```python
from build123d import *

# Parameters (mm, degrees)
SKETCH1_W           = 63.5
SKETCH1_H           = 48.26
BOSS_EXTRUDE1_DEPTH = 6.35
SKETCH2_R           = 3.683
CUT_EXTRUDE1_DEPTH  = 4.318
SKETCH3_R           = 2.159
CUT_EXTRUDE2_DEPTH  = 4.318
SKETCH5_W           = 46.99
SKETCH5_H           = 6.35
CUT_EXTRUDE3_DEPTH  = 2.032
SKETCH4_R           = 1.905
CUT_EXTRUDE4_DEPTH  = 14.732


with BuildPart() as part:
    # Sketch1 → Boss-Extrude1 (new body)
    with BuildSketch(Plane(origin=(0, 0, 0), x_dir=(1, 0, 0), z_dir=(0, 1, 0))):
        Rectangle(SKETCH1_W, SKETCH1_H)
    extrude(amount=-BOSS_EXTRUDE1_DEPTH)

    # Sketch2 → Cut-Extrude1 (cut)
    with BuildSketch(Plane(origin=(0, 0, 0), x_dir=(1, 0, 0), z_dir=(0, 1, 0))):
        with Locations((-19.05, 11.43)):
            Circle(SKETCH2_R)
    cut_extrude1 = extrude(amount=-CUT_EXTRUDE1_DEPTH, mode=Mode.SUBTRACT)

    # Sketch3 → Cut-Extrude2 (cut)
    with BuildSketch(Plane(origin=(0, -4.318, 0), x_dir=(1, 0, 0), z_dir=(0, 1, 0))):
        with Locations((-19.05, 11.43)):
            Circle(SKETCH3_R)
    cut_extrude2 = extrude(amount=-CUT_EXTRUDE2_DEPTH, mode=Mode.SUBTRACT)

    # Sketch5 → Cut-Extrude3 (cut)
    with BuildSketch(Plane.XZ.offset(6.35)):
        with Locations((8.255, 0)):
            Rectangle(SKETCH5_W, SKETCH5_H)
    extrude(amount=-CUT_EXTRUDE3_DEPTH, mode=Mode.SUBTRACT)

    # Sketch4 → Cut-Extrude4 (cut)
    with BuildSketch(Plane(origin=(0, 0, 0), x_dir=(1, 0, 0), z_dir=(0, 1, 0))):
        with Locations((-13.208, -19.558)):
            Circle(SKETCH4_R)
        with Locations((-13.208, 19.442)):
            Circle(SKETCH4_R)
        with Locations((24.638, -19.558)):
            Circle(SKETCH4_R)
        with Locations((24.638, 19.442)):
            Circle(SKETCH4_R)
    extrude(amount=-CUT_EXTRUDE4_DEPTH, mode=Mode.SUBTRACT)

    # Mirror1: Cut-Extrude1, Cut-Extrude2 across plane
    add(cut_extrude1.mirror(Plane.XY), mode=Mode.SUBTRACT)
    add(cut_extrude2.mirror(Plane.XY), mode=Mode.SUBTRACT)


solid = part.part
```
Model file for the job. Use its own axes, mm. A direction names the side the tool comes from. Coordinates: 2 decimals unless noted, no trailing zeros. Order: outer loops, then holes, each group sorted by start corner. A loop starts at its lowest first (then second) coordinate and runs counter-clockwise, first axis right, second up. Notation, with made-up numbers: M 5.25,74 L 24.25,74 A25 ccw 24.25,96 Z; hole C -35.75,4 d1. An arc over 180 degrees is marked long. Answer as CSV lines item,"result".
(1) Flat gauge pins, fed straight in: pin 1 (3 mm diameter, centred on x = 24.638, z = 19.558, fed in from -Y); pin 2 (3 mm diameter, centred on x = 3, z = 0.5, fed in from -Y); pin 3 (2 mm diameter, centred on y = -5.5, z = 1, fed in from +X). Where does each tip first touch, or does it go through?
Geometry says:
pin 1,"passes through"
pin 2,"stops at y = -4.32"
pin 3,"stops at x = -15.24"
(2) Band-saw the part on C-C, the plane z = -2.5. List the corners of the cut face in (x, y), then the cut area to 3 significant figures.
Geometry says:
outline,"M -31.75,-6.35 L -15.24,-6.35 L -15.24,-4.32 L 31.75,-4.32 L 31.75,0 L -31.75,0 Z"
area,"308 mm2"
(3) Band-saw the part on D-D, the plane y = -5.5. List the corners of the cut face in (x, z) (3 decimals), then the cut area to 3 significant figures.
Geometry says:
outline,"M -31.75,-24.13 L 31.75,-24.13 L 31.75,-3.175 L -15.24,-3.175 L -15.24,3.175 L 31.75,3.175 L 31.75,24.13 L -31.75,24.13 Z; hole C -19.05,-11.43 d4.318; hole C -19.05,11.43 d4.318; hole C -13.208,-19.442 d3.81; hole C -13.208,19.558 d3.81; hole C 24.638,-19.442 d3.81; hole C 24.638,19.558 d3.81"
area,"2,690 mm2"
(4) 3-axis set-ups, long thin cutter, end or side, ignore diameter. For faces 1 (the flat face through (-31.75, -3, 0)), 2 (the flat face through (8, -5, -3.175)), 3 (the cylindrical face through (-15.648, -2.129, 10.019)): which of +Z, -Z, +X, -X, +Y, -Y reach the whole face in a straight line?
Geometry says:
face 1,"+Z, -Z, -X, +Y, -Y"
face 2,"+X, -Y"
face 3,"+Y"
(5) Band-saw the part on B-B, the plane z = 11.43. List the corners of the cut face in (x, y), then the cut area to 3 significant figures.
Geometry says:
outline,"M -31.75,-6.35 L -21.21,-6.35 L -21.21,-4.32 L -22.73,-4.32 L -22.73,0 L -31.75,0 Z; M -16.89,-6.35 L 31.75,-6.35 L 31.75,0 L -15.37,0 L -15.37,-4.32 L -16.89,-4.32 Z"
area,"363 mm2"
(6) Pull direction Z, two halves, no side cores. Call faces 4 (the flat face through (0, -3, -24.13)), 5 (the flat face through (-15.24, -5, 0)), 6 (the flat face through (0, 0, 0)): +Z half, -Z half, draft (parallel to the pull), parting line (faces both ways), or undercut.
Geometry says:
face 4,"-Z half"
face 5,"undercut"
face 6,"draft"
(7) Band-saw the part on A-A, the plane x = -19.05. List the corners of the cut face in (y, z).
Geometry says:
outline,"M -6.35,-24.13 L 0,-24.13 L 0,-15.11 L -4.32,-15.11 L -4.32,-13.59 L -6.35,-13.59 Z; M -6.35,-9.27 L -4.32,-9.27 L -4.32,-7.75 L 0,-7.75 L 0,7.75 L -4.32,7.75 L -4.32,9.27 L -6.35,9.27 Z; M -6.35,13.59 L -4.32,13.59 L -4.32,15.11 L 0,15.11 L 0,24.13 L -6.35,24.13 Z"
(8) Wall check: line 1 along Z through (x, y) = (-19.05, -2.15); line 2 along Z through (x, y) = (-19.05, -5.85); line 3 along Z through (x, y) = (3.5, -5.25) (3 decimals). Give the ranges that are in metal, low to high.
Geometry says:
line 1,"z = -24.13 to -15.11, -7.75 to 7.75, 15.11 to 24.13"
line 2,"z = -24.13 to -13.59, -9.27 to 9.27, 13.59 to 24.13"
line 3,"z = -24.13 to -3.175, 3.175 to 24.13"
